Source: CAD feature listing. Evaluate the final solid. Frame: model axes, mm. Face numbers are marked on the shaded views. A direction names the side the tool comes from. Give positions to 0.01 mm unless a question says otherwise; leave off trailing zeros. Order: outer loops, then holes, each group sorted by start corner. A loop starts at its lowest first (then second) coordinate and runs counter-clockwise, first axis right, second up.
1) Section C-C, the plane z = 55. Return loops of the section in (x, y).
2) Access query for the marked faces 1, 2, 3 and 4. Directions: +Z, -Z, +X, -X, +Y, -Y. A direction counts if a zero-diameter tool reaches every point of the face in a straight line with its end or side. Return the directions, or none.
3) Section D-D, the plane z = 6. Return loops of the section in (x, y), plus the area to 3 significant figures.
4) First-contact query: P1, Ø5, axis at x = -3, z = 61, coming from the -Y side; P2, Ø5, axis at x = -9, y = 1, coming from the +Z side; P3, Ø4, axis at y = 17.5, z = 31.5, coming from the -X side. Flat tips, straight axial feed; report the tip coordinate or a pass-through.
5) Section B-B, the plane y = 2. Return loops of the section in (x, z), plus the area to 3 significant figures.
6) Material intervals for line 1 (Z direction, x = 7.5, y = -8.5); line 2 (X direction, y = 22, z = 6.5); line 3 (X direction, y = -18, z = 13.5), sorted ascending.
7) Section A-A, the plane x = -1. Return loops of the section in (y, z).
```python
from build123d import *

# Parameters (mm, degrees)
F1_DEPTH = 30
F3_DEPTH = 40


with BuildPart() as f1:
    # F0 (on Top) → F1 (new body)
    with BuildSketch(Plane.XY):
        Polygon((18.163563, 25), (-18.163563, 25), (-29.389263, -9.54915), (0, -30.901699), (29.389263, -9.54915), align=None)
    extrude(amount=F1_DEPTH)

    # F2 (on face) → F3 (join)
    with BuildSketch(Plane.XY.offset(30)):
        Polygon((-5.877853, -1.90983), (0, -6.18034), (5.877853, -1.90983), (3.632713, 5), (-3.632713, 5), align=None)
    extrude(amount=F3_DEPTH)


solid = f1.part
```
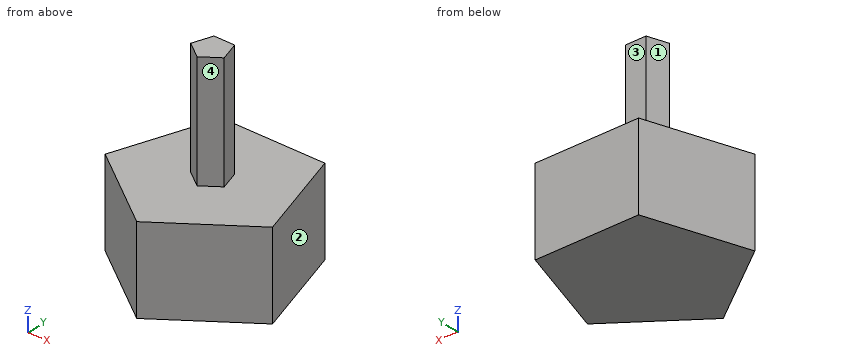
From the geometry:
1. outline: (-5.88, -1.91) - (0, -6.18) - (5.88, -1.91) - (3.63, 5) - (-3.63, 5) - close
2. face 1: +Z, -X, +Y
2. face 2: +Z, -Z, +X, +Y
2. face 3: +Z, +X, -X, +Y
2. face 4: +Z, +X, -Y
3. outline: (-29.39, -9.55) - (0, -30.9) - (29.39, -9.55) - (18.16, 25) - (-18.16, 25) - close
3. area: 2,270 mm2
4. P1: stops at y = -5.82
4. P2: stops at z = 30
4. P3: stops at x = -21.03
5. outline: (-25.64, 0) - (25.64, 0) - (25.64, 30) - (4.61, 30) - (4.61, 70) - (-4.61, 70) - (-4.61, 30) - (-25.64, 30) - close
5. area: 1,910 mm2
6. line 1: z = 0 to 30
6. line 2: x = -19.14 to 19.14
6. line 3: x = -17.76 to 17.76
7. outline: (-30.18, 0) - (25, 0) - (25, 30) - (5, 30) - (5, 70) - (-5.45, 70) - (-5.45, 30) - (-30.18, 30) - close
